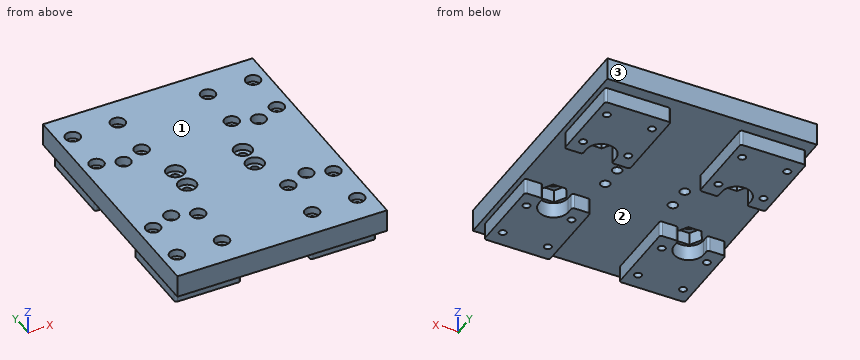
from build123d import *

# Parameters (mm, degrees)
SKETCH_W        = 93
SKETCH_H        = 113
SKETCH_R        = 2.1
SKETCH_R_2      = 1.6
SKETCH_R_3      = 3.2
PAD_DEPTH       = 17
SKETCH001_W     = 93
SKETCH001_H     = 113
POCKET_DEPTH    = 7
SKETCH003_R     = 3.25
POCKET001_DEPTH = 3.2
SKETCH004_R     = 4
POCKET002_DEPTH = 3
POCKET003_DEPTH = 5.7


with BuildPart() as part:
    # Sketch → Pad (new body)
    with BuildSketch(Plane.XY):
        with Locations((46.5, 56.5)):
            Rectangle(SKETCH_W, SKETCH_H)
        with Locations((31.5, 61.5)):
            Circle(SKETCH_R, mode=Mode.SUBTRACT)
        with Locations((61.5, 61.5)):
            Circle(SKETCH_R, mode=Mode.SUBTRACT)
        with Locations((61.5, 51.5)):
            Circle(SKETCH_R, mode=Mode.SUBTRACT)
        with Locations((31.5, 51.5)):
            Circle(SKETCH_R, mode=Mode.SUBTRACT)
        with Locations((6.5, 100.3)):
            Circle(SKETCH_R_2, mode=Mode.SUBTRACT)
        with Locations((26.5, 100.3)):
            Circle(SKETCH_R_2, mode=Mode.SUBTRACT)
        with Locations((26.5, 80.3)):
            Circle(SKETCH_R_2, mode=Mode.SUBTRACT)
        with Locations((6.5, 80.3)):
            Circle(SKETCH_R_2, mode=Mode.SUBTRACT)
        with Locations((26.5, 12.7)):
            Circle(SKETCH_R_2, mode=Mode.SUBTRACT)
        with Locations((6.5, 12.7)):
            Circle(SKETCH_R_2, mode=Mode.SUBTRACT)
        with Locations((6.5, 32.7)):
            Circle(SKETCH_R_2, mode=Mode.SUBTRACT)
        with Locations((26.5, 32.7)):
            Circle(SKETCH_R_2, mode=Mode.SUBTRACT)
        with Locations((66.5, 100.3)):
            Circle(SKETCH_R_2, mode=Mode.SUBTRACT)
        with Locations((86.5, 100.3)):
            Circle(SKETCH_R_2, mode=Mode.SUBTRACT)
        with Locations((86.5, 80.3)):
            Circle(SKETCH_R_2, mode=Mode.SUBTRACT)
        with Locations((66.5, 80.3)):
            Circle(SKETCH_R_2, mode=Mode.SUBTRACT)
        with Locations((66.5, 32.7)):
            Circle(SKETCH_R_2, mode=Mode.SUBTRACT)
        with Locations((86.5, 32.7)):
            Circle(SKETCH_R_2, mode=Mode.SUBTRACT)
        with Locations((86.5, 12.7)):
            Circle(SKETCH_R_2, mode=Mode.SUBTRACT)
        with Locations((66.5, 12.7)):
            Circle(SKETCH_R_2, mode=Mode.SUBTRACT)
        with Locations((16.5, 36.5)):
            Circle(SKETCH_R_3, mode=Mode.SUBTRACT)
        with Locations((76.5, 36.5)):
            Circle(SKETCH_R_3, mode=Mode.SUBTRACT)
        with Locations((76.5, 76.5)):
            Circle(SKETCH_R_3, mode=Mode.SUBTRACT)
        with Locations((16.5, 76.5)):
            Circle(SKETCH_R_3, mode=Mode.SUBTRACT)
    extrude(amount=PAD_DEPTH)

    # Sketch001 (on Face29 of Pad) → Pocket (cut)
    with BuildSketch(Plane(origin=(0, 84, 0), x_dir=(1, 0, 0), z_dir=(0, 0, -1))):
        with Locations((46.5, 27.5)):
            Rectangle(SKETCH001_W, SKETCH001_H)
        with BuildLine():
            Line((2, 45.1), (2, 77.50001))
            ThreePointArc((3, 78.5), (2.292897, 78.20711), (2, 77.50001))
            Line((3, 78.5), (30, 78.5))
            ThreePointArc((31, 77.50001), (30.707103, 78.20711), (30, 78.5))
            Line((31, 77.50001), (31, 45.1))
            ThreePointArc((30, 44.1), (30.707107, 44.392893), (31, 45.1))
            Line((30, 44.1), (24, 44.1))
            ThreePointArc((23, 45.1), (23.292893, 44.392893), (24, 44.1))
            Line((23, 47.5), (23, 45.1))
            ThreePointArc((23, 47.5), (16.5, 54), (10, 47.5))
            Line((10, 47.5), (10, 45.1))
            ThreePointArc((9, 44.1), (9.707107, 44.392893), (10, 45.1))
            Line((3, 44.1), (9, 44.1))
            ThreePointArc((2, 45.1), (2.292893, 44.392893), (3, 44.1))
        make_face(mode=Mode.SUBTRACT)
        with BuildLine():
            ThreePointArc((89.999999, 44.1), (90.707107, 44.392893), (91.000001, 45.1))
            Line((91.000001, 77.5), (91.000001, 45.1))
            ThreePointArc((91.000001, 77.5), (90.707107, 78.207107), (90.000001, 78.5))
            Line((63.000001, 78.5), (90.000001, 78.5))
            ThreePointArc((63.000001, 78.5), (62.292894, 78.207107), (62.000001, 77.5))
            Line((62.000001, 45.1), (62.000001, 77.5))
            ThreePointArc((62.000001, 45.1), (62.292894, 44.392893), (63.000001, 44.1))
            Line((63.000001, 44.1), (69, 44.1))
            ThreePointArc((69, 44.1), (69.707107, 44.392893), (70, 45.1))
            Line((70, 47.5), (70, 45.1))
            ThreePointArc((83, 47.5), (76.5, 54), (70, 47.5))
            Line((83, 47.5), (83, 45.1))
            ThreePointArc((83, 45.1), (83.292893, 44.392893), (84, 44.1))
            Line((89.999999, 44.1), (84, 44.1))
        make_face(mode=Mode.SUBTRACT)
        with BuildLine():
            Line((31, 9.9), (31, -22.5))
            ThreePointArc((30, -23.5), (30.707107, -23.207107), (31, -22.5))
            Line((30, -23.5), (3, -23.5))
            ThreePointArc((2, -22.5), (2.292893, -23.207107), (3, -23.5))
            Line((2, -22.5), (2, 9.9))
            ThreePointArc((3, 10.9), (2.292893, 10.607107), (2, 9.9))
            Line((3, 10.9), (9, 10.9))
            ThreePointArc((10, 9.9), (9.707107, 10.607107), (9, 10.9))
            Line((10, 7.5), (10, 9.9))
            ThreePointArc((10, 7.5), (16.5, 1), (23, 7.5))
            Line((23, 7.5), (23, 9.9))
            ThreePointArc((24, 10.9), (23.292893, 10.607107), (23, 9.9))
            Line((30, 10.9), (24, 10.9))
            ThreePointArc((31, 9.9), (30.707107, 10.607107), (30, 10.9))
        make_face(mode=Mode.SUBTRACT)
        with BuildLine():
            Line((91, 9.9), (91, -22.5))
            ThreePointArc((90, -23.5), (90.707107, -23.207107), (91, -22.5))
            Line((90, -23.5), (63, -23.5))
            ThreePointArc((62, -22.5), (62.292893, -23.207107), (63, -23.5))
            Line((62, -22.5), (62, 9.9))
            ThreePointArc((63, 10.9), (62.292893, 10.607107), (62, 9.9))
            Line((63, 10.9), (69, 10.9))
            ThreePointArc((70, 9.9), (69.707107, 10.607107), (69, 10.9))
            Line((70, 7.5), (70, 9.9))
            ThreePointArc((70, 7.5), (76.5, 1), (83, 7.5))
            Line((83, 7.5), (83, 9.9))
            ThreePointArc((84, 10.9), (83.292893, 10.607107), (83, 9.9))
            Line((90, 10.9), (84, 10.9))
            ThreePointArc((91, 9.9), (90.707107, 10.607107), (90, 10.9))
        make_face(mode=Mode.SUBTRACT)
    extrude(amount=-POCKET_DEPTH, mode=Mode.SUBTRACT)

    # Sketch003 (on Face4 of Pocket) → Pocket001 (cut)
    with BuildSketch(Plane.XY.offset(17)):
        with Locations((6.5, 100.3)):
            Circle(SKETCH003_R)
        with Locations((26.5, 100.3)):
            Circle(SKETCH003_R)
        with Locations((26.5, 80.3)):
            Circle(SKETCH003_R)
        with Locations((6.5, 80.3)):
            Circle(SKETCH003_R)
        with Locations((66.5, 100.3)):
            Circle(SKETCH003_R)
        with Locations((66.5, 80.3)):
            Circle(SKETCH003_R)
        with Locations((86.5, 80.3)):
            Circle(SKETCH003_R)
        with Locations((86.5, 100.3)):
            Circle(SKETCH003_R)
        with Locations((86.5, 12.7)):
            Circle(SKETCH003_R)
        with Locations((66.5, 12.7)):
            Circle(SKETCH003_R)
        with Locations((66.5, 32.7)):
            Circle(SKETCH003_R)
        with Locations((86.5, 32.7)):
            Circle(SKETCH003_R)
        with Locations((6.5, 32.7)):
            Circle(SKETCH003_R)
        with Locations((26.5, 32.7)):
            Circle(SKETCH003_R)
        with Locations((26.5, 12.7)):
            Circle(SKETCH003_R)
        with Locations((6.5, 12.7)):
            Circle(SKETCH003_R)
    extrude(amount=-POCKET001_DEPTH, mode=Mode.SUBTRACT)

    # Sketch004 (on Face4 of Pocket001) → Pocket002 (cut)
    with BuildSketch(Plane.XY.offset(17)):
        with Locations((31.5, 61.5)):
            Circle(SKETCH004_R)
        with Locations((31.5, 51.5)):
            Circle(SKETCH004_R)
        with Locations((61.5, 51.5)):
            Circle(SKETCH004_R)
        with Locations((61.5, 61.5)):
            Circle(SKETCH004_R)
    extrude(amount=-POCKET002_DEPTH, mode=Mode.SUBTRACT)

    # Sketch005 (on Face2 of Pocket002) → Pocket003 (cut)
    with BuildSketch(Plane(origin=(0, 113, 7), x_dir=(1, 0, 0), z_dir=(0, 0, -1))):
        Polygon((10.668762, 36.5), (13.584381, 31.45), (19.415619, 31.45), (22.331238, 36.5), (19.415619, 41.55), (13.584381, 41.55), align=None)
        Polygon((73.584381, 31.45), (79.415619, 31.45), (82.331238, 36.5), (79.415619, 41.55), (73.584381, 41.55), (70.668762, 36.5), align=None)
        Polygon((73.584381, 71.45), (79.415619, 71.45), (82.331238, 76.5), (79.415619, 81.55), (73.584381, 81.55), (70.668762, 76.5), align=None)
        Polygon((13.584381, 71.45), (19.415619, 71.45), (22.331238, 76.5), (19.415619, 81.55), (13.584381, 81.55), (10.668762, 76.5), align=None)
    extrude(amount=-POCKET003_DEPTH, mode=Mode.SUBTRACT)


solid = part.part
Here's how the part is built. I have some questions about the finished solid (model axes, mm). Face numbers are marked on the shaded views. Coordinates: 2 decimals unless noted, no trailing zeros. Order: outer loops, then holes, each group sorted by start corner. A loop starts at its lowest first (then second) coordinate and runs counter-clockwise, first axis right, second up. Notation, with made-up numbers: M -30,65 L -5,65 A15 ccw -5,92 Z; hole C 27.5,-14 d5. An arc over 180 degrees is marked long. Answer as CSV lines item,"result". Start each with the question number.
1. I want a section at D-D, the plane z = 1.75. Count the separate pieces of the cut face and the enclosed holes in it, and give its area (3 significant figures).
2. For pin 1 (5 mm diameter, centred on x = 26.5, y = 100.3, fed in from +Z); pin 2 (5.5 mm diameter, centred on x = 16, z = 2.5, fed in from +Y); pin 3 (1.9 mm diameter, centred on x = 26.5, y = 80.3, fed in from -Z); pin 4 (3.5 mm diameter, centred on x = 76, z = 2, fed in from -Y), each with a flat end and sliding along its axis, tell me the tip position at first contact or that it passes through.
3. We'd pull the mould along Y, two halves only. Please class the marked faces 1, 2 and 3: released by +Y, released by -Y, zero draft, split by the parting line, or undercut.
4. I want a section at A-A, the plane y = 51.5. Write out the boundary of the cut face in (x, z).
5. I need wall thicknesses on line 1 (Y direction, x = 86.5, z = 4.25); line 2 (Y direction, x = 86.5, z = 15.5); line 3 (X direction, y = 36.5, z = 13.6). Which ranges of each line are inside material? Lowest first, please. Write a range as [from, to].
6. I want a section at C-C, the plane y = 89. Write out the boundary of the cut face in (x, z).
7. I want a section at B-B, the plane x = 16.5. Write out the boundary of the cut face in (y, z), and give its area (3 significant figures).
Recorded:
1,separate pieces,"4"
1,enclosed holes,"16"
1,area,"3,410 mm2"
2,pin 1,"stops at z = 13.8"
2,pin 2,"stops at y = 107.5"
2,pin 3,"passes through"
2,pin 4,"stops at y = 5.5"
3,face 1,"zero draft"
3,face 2,"undercut"
3,face 3,"released by +Y"
4,outline,"M 0,7 L 29.4,7 L 29.4,14 L 27.5,14 L 27.5,17 L 0,17 Z; M 33.6,7 L 59.4,7 L 59.4,14 L 57.5,14 L 57.5,17 L 35.5,17 L 35.5,14 L 33.6,14 Z; M 63.6,7 L 93,7 L 93,17 L 65.5,17 L 65.5,14 L 63.6,14 Z"
5,line 1,"y = [5.5, 11.1], [14.3, 31.1], [34.3, 39.9], [73.1, 78.7], [81.9, 98.7], [101.9, 107.5]"
5,line 2,"y = [0, 9.45], [15.95, 29.45], [35.95, 77.05], [83.55, 97.05], [103.55, 113]"
5,line 3,"x = [0, 13.3], [19.7, 73.3], [79.7, 93]"
6,outline,"M 0,7 L 2,7 L 2,0 L 31,0 L 31,7 L 62,7 L 62,0 L 91,0 L 91,7 L 93,7 L 93,17 L 0,17 Z"
7,outline,"M 0,7 L 5.5,7 L 5.5,0 L 30,0 L 30,7 L 31.45,7 L 31.45,12.7 L 33.3,12.7 L 33.3,17 L 0,17 Z; M 39.7,12.7 L 41.55,12.7 L 41.55,7 L 71.45,7 L 71.45,12.7 L 73.3,12.7 L 73.3,17 L 39.7,17 Z; M 79.7,12.7 L 81.55,12.7 L 81.55,7 L 83,7 L 83,0 L 107.5,0 L 107.5,7 L 113,7 L 113,17 L 79.7,17 Z"
7,area,"1,300 mm2"
